```python
from build123d import *

# Parameters (mm, degrees)
F0_W     = 1219.2
F0_H     = 1016
F1_DEPTH = 12.7
F2_W     = 254
F2_H     = 254
F2_W_2   = 304.8
F2_H_2   = 152.4
F3_DEPTH = 133.35
F4_W     = 1219.2
F4_H     = 1016
F5_DEPTH = 12.7
F6_W     = 254
F6_H     = 228.6
F7_DEPTH = 101.6
F8_R     = 63.5
F9_DEPTH = 57.151


with BuildPart() as f1:
    # F0 (on Top) → F1 (new body)
    with BuildSketch(Plane.XY):
        Rectangle(F0_W, F0_H)
    extrude(amount=F1_DEPTH)

    # F2 (on face) → F3 (join)
    with BuildSketch(Plane.XY.offset(12.7)):
        with Locations((-482.6, 381)):
            Rectangle(F2_W, F2_H)
        with Locations((482.6, 381)):
            Rectangle(F2_W, F2_H)
        with Locations((482.6, -381)):
            Rectangle(F2_W, F2_H)
        with Locations((-482.6, -381)):
            Rectangle(F2_W, F2_H)
        with Locations((0, 381)):
            Rectangle(F2_W_2, F2_H)
        with Locations((0, -381)):
            Rectangle(F2_W_2, F2_H)
        with Locations((482.6, 0)):
            Rectangle(F2_W, F2_H_2)
        with Locations((-482.6, 0)):
            Rectangle(F2_W, F2_H_2)
        Rectangle(F2_W_2, F2_H_2)
    extrude(amount=F3_DEPTH)

    # F4 (on face) → F5 (join)
    with BuildSketch(Plane.XY.offset(146.05)):
        Rectangle(F4_W, F4_H)
    extrude(amount=F5_DEPTH)

    # F6 (on face) → F7 (cut)
    with BuildSketch(Plane.XY.offset(158.75)):
        with Locations((0, 393.7)):
            Rectangle(F6_W, F6_H)
    extrude(amount=-F7_DEPTH, mode=Mode.SUBTRACT)

    # F8 (on face) → F9 (cut, through all)
    with BuildSketch(Plane.XY.offset(57.15)):
        with Locations((0, 393.7)):
            Circle(F8_R)
    extrude(amount=-F9_DEPTH, mode=Mode.SUBTRACT)


solid = f1.part
```
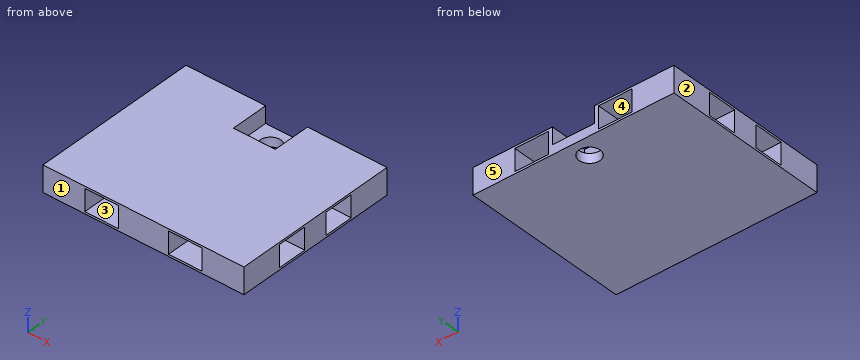
Could you check a few things on this model? Use its own coordinates, in mm. Face numbers are marked on the shaded views. A direction names the side the tool comes from. Round coordinates to 2 decimals unless told otherwise and drop trailing zeros. Loops run counter-clockwise (first coordinate to the right, second up) from the corner with the lowest first, then second, coordinate; pieces in that order, holes last. Notation, with made-up numbers: (-11, 10.25) - (-7, 10.25) arc R15 cw to (-7, 37.25) - close; hole circle Ø9 at (-1.5, 10.25). An arc over 180 degrees is marked (long way). Answer in a Markdown table with one row per item. Add a question column.
(1) For the marked faces 4 and 5, which set-ups out of +Z, -Z, +X, -X, +Y, -Y let a thin tool reach every point of the face, with its end or its side?
(2) If we section it at C-C (x = 0): Please give me the cut outline in (y, z).
(3) If we mould it in two halves opening along X, with no side actions, what happens to the marked faces 1, 2 and 3? For each: pulls with the +X half, pulls with the -X half, needs draft (parallel to the pull), parting line crosses it, or undercut.
(4) If we section it at D-D (y = -134.5): Please give me the cut outline in (x, z).
(5) I need wall thicknesses on line 1 along X through (y, z) = (393, 26); line 2 along X through (y, z) = (-29, 33); line 3 along Y through (x, z) = (0, 36.5). Which ranges of each line are inside material? Lowest first, please.
(6) If we section it at A-A (y = 393.7): Please give me the cut outline in (x, z), plus the area to 3 significant figures.
(7) I'm going to push flat-ended pins straight in: pin 1 (2 mm diameter, centred on x = -62.5, y = -357, fed in from -Z); pin 2 (10 mm diameter, centred on y = -214, z = 22, fed in from +X). Where does each tip first touch, or does it pass through?
(8) If we section it at B-B (x = -380): Please give me the cut outline in (y, z).
Model answer:
| question | item | result |
|---|---|---|
| 1 | face 4 | none |
| 1 | face 5 | +Z, -Z, +X, -X, +Y |
| 2 | outline | (-508, 0) - (330.2, 0) - (330.2, 57.15) - (279.4, 57.15) - (279.4, 158.75) - (-508, 158.75) - close; (457.2, 0) - (508, 0) - (508, 57.15) - (457.2, 57.15) - close; hole (-254, 12.7) - (-76.2, 12.7) - (-76.2, 146.05) - (-254, 146.05) - close; hole (76.2, 12.7) - (254, 12.7) - (254, 146.05) - (76.2, 146.05) - close |
| 3 | face 1 | needs draft |
| 3 | face 2 | pulls with the -X half |
| 3 | face 3 | undercut |
| 4 | outline | (-609.6, 0) - (609.6, 0) - (609.6, 12.7) - (-609.6, 12.7) - close; (-609.6, 146.05) - (609.6, 146.05) - (609.6, 158.75) - (-609.6, 158.75) - close |
| 5 | line 1 | x = -609.6 to -355.6, -152.4 to -63.5, 63.5 to 152.4, 355.6 to 609.6 |
| 5 | line 2 | x = -609.6 to -355.6, -152.4 to 152.4, 355.6 to 609.6 |
| 5 | line 3 | y = -508 to -254, -76.2 to 76.2, 254 to 330.2, 457.2 to 508 |
| 6 | outline | (-609.6, 0) - (-63.5, 0) - (-63.5, 57.15) - (-127, 57.15) - (-127, 158.75) - (-609.6, 158.75) - close; (63.5, 0) - (609.6, 0) - (609.6, 158.75) - (127, 158.75) - (127, 57.15) - (63.5, 57.15) - close; hole (-355.6, 12.7) - (-152.4, 12.7) - (-152.4, 146.05) - (-355.6, 146.05) - close; hole (152.4, 12.7) - (355.6, 12.7) - (355.6, 146.05) - (152.4, 146.05) - close |
| 6 | area | 106,000 mm² |
| 7 | pin 1 | stops at z = 0 |
| 7 | pin 2 | passes through |
| 8 | outline | (-508, 0) - (508, 0) - (508, 158.75) - (-508, 158.75) - close; hole (-254, 12.7) - (-76.2, 12.7) - (-76.2, 146.05) - (-254, 146.05) - close; hole (76.2, 12.7) - (254, 12.7) - (254, 146.05) - (76.2, 146.05) - close |
